Solid Edge part; units mm, degrees
sketch "Sketch1" plane through (0, 0, 0) normal (0, -1, 0) x (1, 0, 0)
  line L0 (6, -6) -> (-6, -6)
  line L1 (-6, -6) -> (-6, 6)
  line L2 (-6, 6) -> (6, 6)
  line L3 (6, 6) -> (6, -6)
  dimension "D1" = 6
  dimension "D2" = 6
extrude "Protrusion1" add sketch "Sketch1" along normal mid plane 12
sketch "Sketch2" plane through (0, 0, 0) normal (0, -1, 0) x (1, 0, 0)
  line L0 (9.56, 3.8003) -> (5.75, 6)
  line L1 (5.75, 6) -> (12.1, 6)
  line L2 (12.1, 6) -> (12.1, -6)
  line L3 (12.1, -6) -> (5.75, -6)
  line L4 (5.75, -6) -> (9.56, -3.8003)
  line L5 (9.56, -3.8003) -> (9.56, 3.8003)
revolve "RevolvedCutout1" cut sketch "Sketch2" angle 360 about axis through (0, 0, 0) along (0, 0, 1)
sketch "Sketch3" plane through (0, 0, 0) normal (1, 0, 0) x (0, 1, 0)
  circle A0 centre (0, 0) radius 2.25
extrude "ExtrudedProtrusion_3" add sketch "Sketch3" along normal mid plane 24
sketch "Sketch4" plane through (0, 0, 0) normal (0, -1, 0) x (1, 0, 0)
  circle A0 centre (0, 0) radius 2.25
extrude "ExtrudedProtrusion_4" add sketch "Sketch4" along normal mid plane 24
fillet "Round_1" radius 0.5 6 edges at (-2.25, -12, 0) (12, -2.25, 0) (-2.25, 12, 0) (-12, -2.25, 0) (-5.75, 0, 6) (-5.75, 0, -6)
extrude "ExtrudedCutout_1" [suppressed]
Work out the finished part from the listing and answer in its coordinate system (mm). A direction names the side the tool comes from. Coordinates: 2 decimals unless noted, no trailing zeros. Write each loop counter-clockwise with the first axis right and the second up, starting at its lowest first coordinate (ties: lowest second). Pieces come first, ordered by that corner, then holes.
Q1. A cutting plane is placed at D-D, the plane x = 10.25. Give the vertices of the cut face in (y, z), then the cut area to 3 significant figures.
Q2. This flat-tipped pin is pushed along its axis until it touches: pin 1 Ø1 at (x, y) = (-7, -0.5) entering from +Z. Where does it stop, or does it pass through?
Q3. A cutting plane is placed at C-C, the plane z = 3.75. Give the vertices of the cut face in (x, y).
Q4. Which of the six approach directions +Z, -Z, +X, -X, +Y, -Y give full straight-line access (tool end or side, diameter ignored) to faces 1 (the face through (-6, 0, 3)), 2 (the face through (-0.29, -8.71, -2.23)), 3 (the face through (6, 0, -3))?
Q5. A cutting plane is placed at A-A, the plane y = 0. Give the vertices of the cut face in (x, z), then the cut area to 3 significant figures.
Q6. Find the intervals of material crossed by line 1 (X direction, y = -2, z = 3.75); line 2 (Z direction, x = -3.5, y = 4.5), in increasing order.
Findings below:
1. outline: circle Ø4.5 at (0, 0)
1. area: 15.9 mm2
2. pin 1: stops at z = 2.25
3. outline: (-6, -6) - (6, -6) - (6, 6) - (-6, 6) - close
4. face 1: -X
4. face 2: -Y
4. face 3: +X
5. outline: (-12, -1.75) arc R0.5 ccw to (-11.5, -2.25) - (-6, -2.25) - (-6, -5.86) - (-5.87, -5.93) arc R0.5 ccw to (-5.62, -6) - (5.62, -6) arc R0.5 ccw to (5.87, -5.93) - (6, -5.86) - (6, -2.25) - (11.5, -2.25) arc R0.5 ccw to (12, -1.75) - (12, 1.75) arc R0.5 ccw to (11.5, 2.25) - (6, 2.25) - (6, 5.86) - (5.87, 5.93) arc R0.5 ccw to (5.62, 6) - (-5.62, 6) arc R0.5 ccw to (-5.87, 5.93) - (-6, 5.86) - (-6, 2.25) - (-11.5, 2.25) arc R0.5 ccw to (-12, 1.75) - close
5. area: 198 mm2
6. line 1: x = -6 to 6
6. line 2: z = -5.99 to 5.99
